from build123d import *
from build123d import SkipClean  # not in build123d's __all__

# Parameters (mm, degrees)
F1_DEPTH      = 72.39
F1_DEPTH_BACK = 50.8
F2_R          = 7.747
F3_DEPTH      = 69.85
F3_DEPTH_BACK = 69.85
F4_W          = 124.6
F4_H          = 26.092820323
F5_DEPTH      = 72.391
F5_DEPTH_BACK = 50.801
F7_DEPTH      = 81.776
F7_DEPTH_BACK = 81.776


with BuildPart() as f1:
    # F0 (on Front) → F1 (new body, two sides)
    with BuildSketch(Plane.XZ) as f1_sk:
        Polygon((80.575, -36.195), (0, -36.195), (-80.575, -36.195), (-80.575, 42.545), (-62.3, 53.0960761694), (-62.3, 79.1888964925), (-63.5, 79.1888964925), (-63.5, 53.7888964925), (-81.775, 43.237820323), (-81.775, -37.395), (0, -37.395), (81.775, -37.395), (81.775, 43.237820323), (63.5, 53.7888964925), (63.5, 79.1888964925), (62.3, 79.1888964925), (62.3, 53.0960761694), (80.575, 42.545), align=None)
    extrude(amount=-F1_DEPTH)
    extrude(f1_sk.sketch, amount=F1_DEPTH_BACK)

    # F2 (on Right) → F3 (join, two sides)
    with BuildSketch(Plane.YZ) as f3_sk:
        with Locations((0, 71.4418964925)):
            Circle(F2_R)
    extrude(amount=-F3_DEPTH)
    extrude(f3_sk.sketch, amount=F3_DEPTH_BACK)

    # F4 (on Front) → F5 (cut, two sides)
    with BuildSketch(Plane.XZ) as f5_sk:
        with Locations((0, 66.142486331)):
            Rectangle(F4_W, F4_H)
    extrude(amount=-F5_DEPTH, mode=Mode.SUBTRACT)
    extrude(f5_sk.sketch, amount=F5_DEPTH_BACK, mode=Mode.SUBTRACT)

    # F6 (on Right) → F7 (cut, two sides)
    with BuildSketch(Plane.YZ) as f7_sk:
        with BuildLine():
            Line((-50.8, 81.7288964925), (-50.8, 31.5978089602))
            Line((-50.8, 31.5978089602), (-5.4779562339, 76.9198527263))
            ThreePointArc((-5.4779562339, 76.9198527263), (0, 79.1888964925), (5.4779562339, 76.9198527263))
            Line((5.4779562339, 76.9198527263), (72.39, 10.0078089602))
            Line((72.39, 10.0078089602), (72.39, 81.7288964925))
            Line((72.39, 81.7288964925), (-50.8, 81.7288964925))
        make_face()
    with SkipClean():  # cleaning this boolean's faces spoils the solid; the shape is the same uncleaned
        extrude(amount=-F7_DEPTH, mode=Mode.SUBTRACT)
        extrude(f7_sk.sketch, amount=F7_DEPTH_BACK, mode=Mode.SUBTRACT)


solid = f1.part
Model file for the job. Use its own axes, mm. A direction names the side the tool comes from. Give positions to 0.01 mm unless a question says otherwise; leave off trailing zeros. Order: outer loops, then holes, each group sorted by start corner. A loop starts at its lowest first (then second) coordinate and runs counter-clockwise, first axis right, second up. Notation, with made-up numbers: (62, 65) - (96, 65) arc R24 cw to (96, 104) - close; hole circle Ø2 at (57.25, -3). An arc over 180 degrees is marked (long way). One line per item, written item: value.
Item 1: Slice it at A-A (z = -2.5). List the corners of the cut face in (x, y) (3 decimals).
Response values:
outline: (-81.775, -50.8) - (-80.575, -50.8) - (-80.575, 72.39) - (-81.775, 72.39) - close; (80.575, -50.8) - (81.775, -50.8) - (81.775, 72.39) - (80.575, 72.39) - close
Item 2: Slice it at D-D (y = 58). List the corners of the cut face in (x, z) (3 decimals), then the cut area to 3 significant figures.
Response values:
outline: (-81.775, -37.395) - (81.775, -37.395) - (81.775, 24.398) - (80.575, 24.398) - (80.575, -36.195) - (-80.575, -36.195) - (-80.575, 24.398) - (-81.775, 24.398) - close
area: 342 mm2
Item 3: Slice it at C-C (x = -27). List the corners of the cut face in (y, z) (3 decimals).
Response values:
outline: (-50.8, -37.395) - (72.39, -37.395) - (72.39, -36.195) - (-50.8, -36.195) - close
Item 4: Tool access for faces 4 (the flat face through (62.3, 0, 63)), 5 (the flat face through (-69.85, 0, 72)), 6 (the flat face through (-80.575, 12, 3)): list every direction of +Z, -Z, +X, -X, +Y, -Y with a clear straight run to the whole face (end or side of a thin tool).
Response values:
face 4: +Z, +Y, -Y
face 5: +Z, -X, +Y, -Y
face 6: +Y, -Y
Item 5: Slice it at B-B (y = -33.5). List the corners of the cut face in (x, z) (3 decimals).
Response values:
outline: (-81.775, -37.395) - (81.775, -37.395) - (81.775, 43.238) - (71.972, 48.898) - (69.572, 48.898) - (80.575, 42.545) - (80.575, -36.195) - (-80.575, -36.195) - (-80.575, 42.545) - (-69.572, 48.898) - (-71.972, 48.898) - (-81.775, 43.238) - close
Item 6: Pin check, flat tips, straight feed: pin 1 Ø13 at (y, z) = (-13.5, 66) entering from -X; pin 2 Ø7 at (y, z) = (-3.5, 60) entering from +X; pin 3 Ø7.5 at (y, z) = (3, 74.5) entering from -X. Stop position of each tip, or through.
Response values:
pin 1: x = -63.5
pin 2: x = 63.5
pin 3: x = -69.85
Item 7: Two-plate mould, pull along Z, no slides. Class faces 1 (the flat face through (-74.9, 36.3, 46.1)), 2 (the flat face through (-62.3, 0, 63)), 3 (the flat face through (63.5, 0, 60)): released by +Z, released by -Z, zero draft, split by the parting line, or undercut.
Response values:
face 1: released by +Z
face 2: zero draft
face 3: undercut
Item 8: Wall check: line 1 (X direction, y = -23, z = 38) (3 decimals); line 2 (X direction, y = -7.5, z = 72); line 3 (Z direction, x = 61.5, y = -36) (3 decimals). Give the ranges that are in metal, low to high.
Response values:
line 1: -81.775 to -80.575, 80.575 to 81.775
line 2: -69.85 to -62.3, 62.3 to 69.85
line 3: -37.395 to -36.195
